The listing builds one solid part. Answer for the finished solid, in the listing's coordinates (mm). Face numbers are marked on the shaded views. Coordinates: 2 decimals unless noted, no trailing zeros. Write each loop counter-clockwise with the first axis right and the second up, starting at its lowest first coordinate (ties: lowest second). Pieces come first, ordered by that corner, then holes.
(1) Given P1, Ø5, axis at y = 12.5, z = -5, coming from the -X side; P2, Ø4, axis at x = 34.5, y = 2.5, coming from the +Z side; P3, Ø3, axis at x = -2.5, y = 1.5, coming from the +Z side; P4, Ø2, axis at x = -32, z = -18, coming from the -Y side, each flat-ended and moving along its own axis, determine where each tip first touches the part or whether it passes through.
(2) Straight lines are drawn through the part: line 1 (X direction, y = 11.5, z = 0); line 2 (Y direction, x = 32, z = -18.5); line 3 (X direction, y = 8.25, z = -37.5). For each, find the intervals that lie inside material, in ascending order.
(3) The part is cut by section C-C on y = 9.75. Determine the outline of the cut face in (x, z), plus the area to 3 significant figures.
(4) The part is cut by section A-A on z = 0. Determine the outline of the cut face in (x, y), plus the area to 3 significant figures.
(5) For a pull along Z with two mould halves and no side action, classify the marked faces 1, 2, 3 and 4 as +Z half, -Z half, draft (parallel to the pull), parting line (faces both ways), or undercut.
(6) The part is cut by section B-B on x = 0. Determine the outline of the cut face in (y, z).
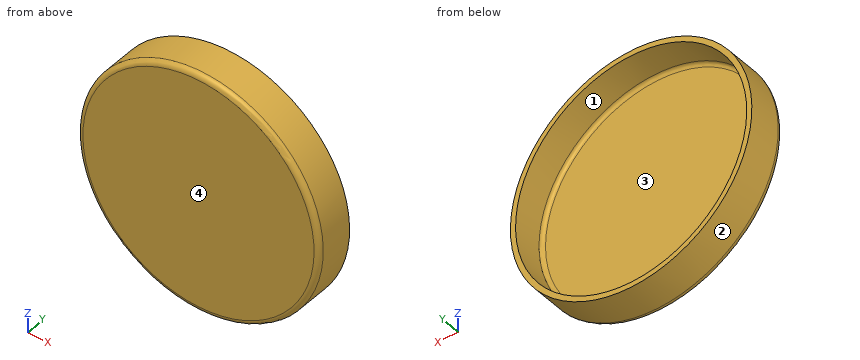
from build123d import *


with BuildPart() as part:
    # Croquis1 → Revolución1 (revolve)
    with BuildSketch(Plane.XY, mode=Mode.PRIVATE) as revoluci_n1_sk:
        with BuildLine():
            Line((45, 0), (0, 0))
            Line((0, 0), (0, 2))
            Line((0, 2), (43.585786438, 2))
            ThreePointArc((43.585786438, 2), (44.585786438, 2.414213562), (45, 3.414213562))
            Line((45, 3.414213562), (45, 15))
            Line((45, 15), (47, 15))
            Line((47, 15), (47, 2))
            ThreePointArc((47, 2), (46.414213562, 0.585786438), (45, 0))
        make_face()
    revolve(revoluci_n1_sk.sketch.rotate(Axis((0, 0, 0), (0, 1, 0)), 90), axis=Axis((0, 0, 0), (0, 1, 0)))


solid = part.part
Model answer:
1. P1: stops at x = -46.93
1. P2: stops at z = 33.95
1. P3: stops at z = 46.99
1. P4: stops at y = 0
2. line 1: x = -47 to -45, 45 to 47
2. line 2: y = 0 to 2
2. line 3: x = -28.33 to -24.87, 24.87 to 28.33
3. outline: circle Ø94 at (0, 0); hole circle Ø90 at (0, 0)
3. area: 578 mm2
4. outline: (-47, 2) arc R2 ccw to (-45, 0) - (45, 0) arc R2 ccw to (47, 2) - (47, 15) - (45, 15) - (45, 3.41) arc R1.41 cw to (43.59, 2) - (-43.59, 2) arc R1.41 cw to (-45, 3.41) - (-45, 15) - (-47, 15) - close
4. area: 239 mm2
5. face 1: undercut
5. face 2: parting line
5. face 3: undercut
5. face 4: draft
6. outline: (0, -45) arc R2 ccw to (2, -47) - (15, -47) - (15, -45) - (3.41, -45) arc R1.41 cw to (2, -43.59) - (2, 43.59) arc R1.41 cw to (3.41, 45) - (15, 45) - (15, 47) - (2, 47) arc R2 ccw to (0, 45) - close
